from build123d import *

# Parameters (mm, degrees)
F1_DEPTH = 3


with BuildPart() as f1:
    # F0 (on Top) → F1 (new body)
    with BuildSketch(Plane.XY):
        with BuildLine():
            ThreePointArc((-75, -110), (0, -132.956233), (75, -110))
            Line((75, -110), (67, -110))
            Line((67, -110), (67, -27.5))
            Line((67, -27.5), (75, -27.5))
            Line((75, -27.5), (75, 15.416617))
            Line((75, 15.416617), (67, 15.416617))
            Line((67, 15.416617), (67, 97.916617))
            Line((67, 97.916617), (75, 97.916617))
            ThreePointArc((75, 97.916617), (73.957089, 104.290688), (70.937122, 110))
            ThreePointArc((70.937122, 110), (67.582857, 113.462411), (63.497547, 116.021636))
            ThreePointArc((63.497547, 116.021636), (0, 130.181802), (-63.497547, 116.021636))
            ThreePointArc((-63.497547, 116.021636), (-67.582857, 113.462411), (-70.937122, 110))
            ThreePointArc((-70.937122, 110), (-73.957089, 104.290688), (-75, 97.916617))
            Line((-75, 97.916617), (-67, 97.916617))
            Line((-67, 97.916617), (-67, 15.416617))
            Line((-67, 15.416617), (-75, 15.416617))
            Line((-75, 15.416617), (-75, -27.5))
            Line((-75, -27.5), (-67, -27.5))
            Line((-67, -27.5), (-67, -110))
            Line((-67, -110), (-75, -110))
        make_face()
    extrude(amount=F1_DEPTH)


solid = f1.part
Can you work these out from the model? Positions are in its coordinate system, mm. Round coordinates to 2 decimals unless told otherwise and drop trailing zeros. Loops run counter-clockwise (first coordinate to the right, second up) from the corner with the lowest first, then second, coordinate; pieces in that order, holes last. Notation, with made-up numbers: (-16, 34) - (-3, 34) arc R26 cw to (-3, 68) - close; hole circle Ø2 at (-3, 16). An arc over 180 degrees is marked (long way). Answer in a Markdown table with one row per item. Add a question column.
Q1. I want a section at A-A on z = 1.3. List the corners of the cut face in (x, y) for me.
Q2. I want a section at C-C on x = 28.5. List the corners of the cut face in (y, z) for me.
Q3. I want a section at B-B on y = -76. List the corners of the cut face in (x, z) for me, and give its area (3 significant figures).
Q4. For pin 1 Ø1.5 at (x, z) = (69.5, 2) entering from -Y; pin 2 Ø0.9 at (y, z) = (-52, 2) entering from -X; pin 3 Ø1.5 at (y, z) = (-83.5, 1) entering from +X; pin 4 Ø6 at (x, y) = (-44, -3) entering from -Z, each with a flat end and sliding along its axis, tell me the tip position at first contact or that it passes through.
Q5. I need wall thicknesses on L1, parallel to X at y = 92.5, z = 2; L2, parallel to Y at x = -1, z = 2.1; L3, parallel to Y at x = -52.5, z = 0.95. Which ranges of each line are inside material? Lowest first, please.
A:
| question | item | result |
|---|---|---|
| 1 | outline | (-75, -110) arc R133.99 ccw to (75, -110) - (67, -110) - (67, -27.5) - (75, -27.5) - (75, 15.42) - (67, 15.42) - (67, 97.92) - (75, 97.92) arc R20 ccw to (70.94, 110) arc R20 ccw to (63.5, 116.02) arc R149.45 ccw to (-63.5, 116.02) arc R20 ccw to (-70.94, 110) arc R20 ccw to (-75, 97.92) - (-67, 97.92) - (-67, 15.42) - (-75, 15.42) - (-75, -27.5) - (-67, -27.5) - (-67, -110) - close |
| 2 | outline | (-129.89, 0) - (127.44, 0) - (127.44, 3) - (-129.89, 3) - close |
| 3 | outline | (-67, 0) - (67, 0) - (67, 3) - (-67, 3) - close |
| 3 | area | 402 mm^2 |
| 4 | pin 1 | y = -113.97 |
| 4 | pin 2 | x = -67 |
| 4 | pin 3 | x = 67 |
| 4 | pin 4 | z = 0 |
| 5 | L1 | -67 to 67 |
| 5 | L2 | -132.95 to 130.18 |
| 5 | L3 | -122.24 to 120.66 |
